The drawing under review shows one solid part. Ordinate dimensions are in mm from its lowest x, y, z. Round coordinates to 2 decimals unless told otherwise and drop trailing zeros. Write each loop counter-clockwise with the first axis right and the second up, starting at its lowest first coordinate (ties: lowest second). Pieces come first, ordered by that corner, then holes. Notation, with made-up numbers: (43, -33) -> (75, -33) arc R26 ccw to (75, -5) -> close; hole circle Ø3 at (80, 11). An arc over 180 degrees is marked (long way). Write item = value, one per line. Start each with the question number.
Item 1: To check wall thickness, follow L1, parallel to Y at x = 35.2, z = 2.5; L2, parallel to Y at x = 24.5, z = 1.5 (1 decimal); L3, parallel to Y at x = 22.5, z = 2.25. State the ranges of each line that lie inside material, in increasing order.
Item 2: Add section A-A, the plane x = 9.8. State the section outline as (y, z) points.
Item 3: Add section C-C, the plane x = 22.5. State the section outline as (y, z) points.
Item 4: Add section B-B, the plane z = 1. State how many separate pieces and enclosed holes the cut face has, then the cut area to 3 significant figures.
Item 5: For pin 1 Ø1.9 at (x, y) = (7.5, 37) entering from -Z, flat-tipped, find the tip position at first contact; note if it passes through.
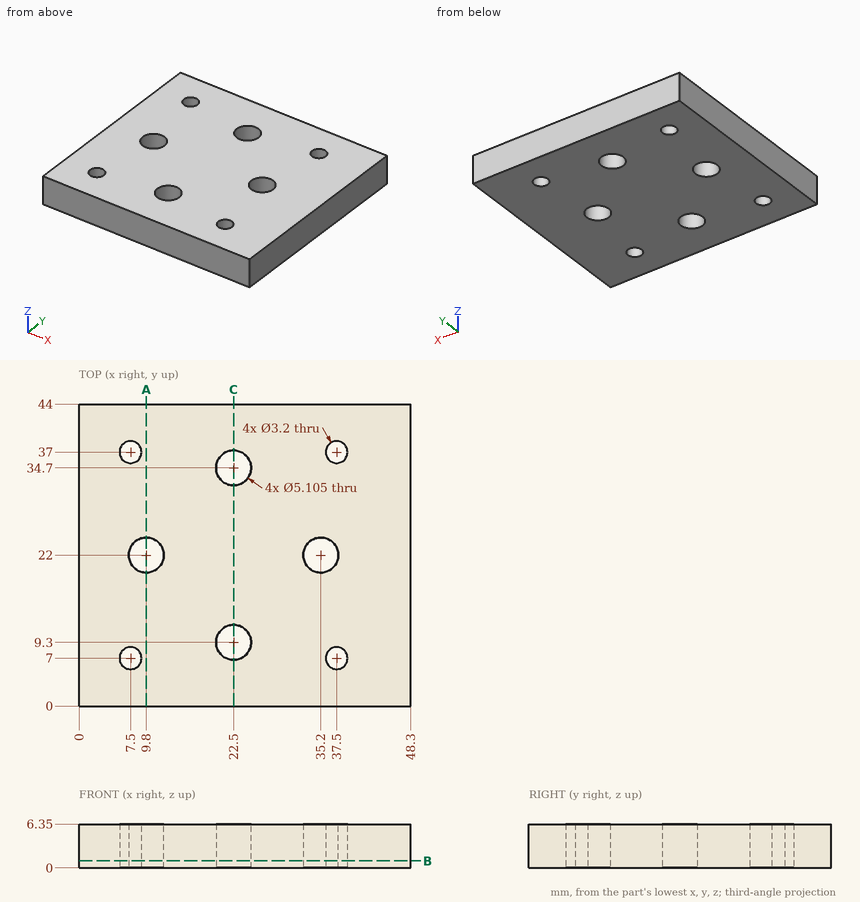
Result set:
q1.L1 = 0 to 19.45, 24.55 to 44
q1.L2 = 0 to 7.7, 10.9 to 33.1, 36.3 to 44
q1.L3 = 0 to 6.75, 11.85 to 32.15, 37.25 to 44
q2.outline = (0, 0) -> (19.45, 0) -> (19.45, 6.35) -> (0, 6.35) -> close; (24.55, 0) -> (44, 0) -> (44, 6.35) -> (24.55, 6.35) -> close
q3.outline = (0, 0) -> (6.75, 0) -> (6.75, 6.35) -> (0, 6.35) -> close; (11.85, 0) -> (32.15, 0) -> (32.15, 6.35) -> (11.85, 6.35) -> close; (37.25, 0) -> (44, 0) -> (44, 6.35) -> (37.25, 6.35) -> close
q4.separate_pieces = 1
q4.enclosed_holes = 8
q4.area = 2,010 mm²
q5.pin_1 = through
